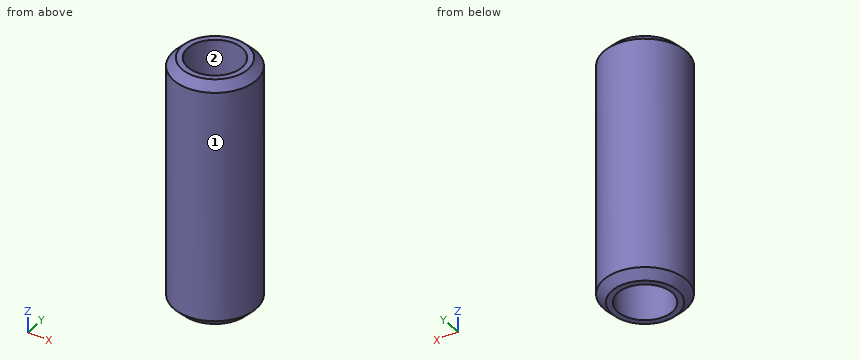
from build123d import *

# Parameters (mm, degrees)
ESQUISSE1_R       = 2.5
EXTRUSION1_DEPTH  = 15
CHANFREIN1_SIZE   = 0.5
TROU_TARAUD_M41_D = 3.3


with BuildPart() as part:
    # Esquisse1 → Extrusion1 (new body)
    with BuildSketch(Plane.XY):
        Circle(ESQUISSE1_R)
    extrude(amount=EXTRUSION1_DEPTH)

    # Chanfrein1
    chanfrein1_edges = [part.edges().sort_by_distance(p)[0] for p in [
        (-2.5, 0, 0),
        (-2.5, 0, 15),
    ]]
    chamfer(chanfrein1_edges, length=CHANFREIN1_SIZE)

    # Trou taraudé M41 (through all)
    with Locations(Plane.XY.offset(15)):
        with Locations((0, 0)):
            Hole(TROU_TARAUD_M41_D / 2)


solid = part.part
Work out the finished part from the listing and answer in its coordinate system (mm). Face numbers are marked on the shaded views. Round coordinates to 2 decimals unless told otherwise and drop trailing zeros. Loops run counter-clockwise (first coordinate to the right, second up) from the corner with the lowest first, then second, coordinate; pieces in that order, holes last. Notation, with made-up numbers: (-18.75, -7.75) - (31.25, -7.75) arc R24 ccw to (31.25, 18.25) - close; hole circle Ø3 at (57, 53.5). An arc over 180 degrees is marked (long way). Use one line per item in the form item = value. Start each with the question number.
(1) Find section A-A on y = 0. Determine the outline of the cut face in (x, z).
(2) Consider line 1 (Y direction, x = 0, z = 10.5); line 2 (X direction, y = 0.15, z = 12); line 3 (X direction, y = -1.35, z = 10.5). Determine where each line is inside the solid, lowest interval first.
(3) Find section C-C on z = 12. Determine the outline of the cut face in (x, y).
(4) Determine the mould class of the marked faces 1 and 2 for opening direction X: +X half, -X half, draft (parallel to the pull), parting line (faces both ways), or undercut.
Answer list:
q1.outline = (-2.5, 0.5) - (-2, 0) - (-1.65, 0) - (-1.65, 15) - (-2, 15) - (-2.5, 14.5) - close; (1.65, 0) - (2, 0) - (2.5, 0.5) - (2.5, 14.5) - (2, 15) - (1.65, 15) - close
q2.line_1 = -2.5 to -1.65, 1.65 to 2.5
q2.line_2 = -2.5 to -1.64, 1.64 to 2.5
q2.line_3 = -2.1 to -0.95, 0.95 to 2.1
q3.outline = circle Ø5 at (0, 0); hole circle Ø3.3 at (0, 0)
q4.face_1 = parting line
q4.face_2 = undercut
